Work out the finished part from the listing and answer in its coordinate system (mm). A direction names the side the tool comes from. Give positions to 0.01 mm unless a question says otherwise; leave off trailing zeros. Loops run counter-clockwise (first coordinate to the right, second up) from the corner with the lowest first, then second, coordinate; pieces in that order, holes last. Notation, with made-up numbers: (-38.75, 42) - (12.25, 42) arc R10 ccw to (12.25, 56) - close; hole circle Ø10 at (74.5, 33.5). An arc over 180 degrees is marked (long way). Use CSV: the item, a comma, the result in double quotes.
from build123d import *

# Parameters (mm, degrees)
F1_DEPTH = 600
F2_R     = 80
F3_DEPTH = 1321.7481718788
F5_DEPTH = 200.001
F6_DEPTH = 200.001


# Not quite as in the source:
# - a feature names something its author has since deleted; it is built from what else it names


with BuildPart() as f1:
    # F0 (on Front) → F1 (new body)
    with BuildSketch(Plane.XZ):
        with BuildLine():
            Line((506.8030357361, -100), (506.8030357361, 300))
            Line((506.8030357361, 300), (292.5279319286, 300))
            ThreePointArc((292.5279319286, 300), (-7.4720680714, 0), (-307.4720680714, 300))
            Line((-307.4720680714, 300), (-521.7471718788, 300))
            Line((-521.7471718788, 300), (-521.7471718788, -100))
            Line((-521.7471718788, -100), (-800, -100))
            Line((-800, -100), (-800, -300))
            Line((-800, -300), (800, -300))
            Line((800, -300), (800, -100))
            Line((800, -100), (506.8030357361, -100))
        make_face()
    extrude(amount=F1_DEPTH)

    # F2 (on face) → F3 (cut, through all)
    with BuildSketch(Plane(origin=(-521.7471718788, 0, 0), x_dir=(0, -1, 0), z_dir=(-1, 0, 0))):
        with Locations((287.7135872841, 150)):
            Circle(F2_R)
    extrude(amount=-F3_DEPTH, mode=Mode.SUBTRACT)

    # F4 (on face) → F5 (cut, through all)
    with BuildSketch(Plane.XY.offset(-100)):
        with BuildLine():
            Line((-610.4801893234, -509.8910629749), (-610.4801893234, -165.6369864941))
            Line((-610.4801893234, -165.6369864941), (-616.1602163315, -165.6369864941))
            ThreePointArc((-616.1602163315, -165.6369864941), (-676.1602163315, -105.6369864941), (-736.1602163315, -165.6369864941))
            Line((-736.1602163315, -165.6369864941), (-741.8402433395, -165.6369864941))
            Line((-741.8402433395, -165.6369864941), (-741.8402433395, -509.8910629749))
            Line((-741.8402433395, -509.8910629749), (-736.1602163315, -509.8910629749))
            ThreePointArc((-736.1602163315, -509.8910629749), (-676.1602163315, -569.8910629749), (-616.1602163315, -509.8910629749))
            Line((-616.1602163315, -509.8910629749), (-610.4801893234, -509.8910629749))
        make_face()
        with BuildLine():
            Line((704.2353129387, -496.3020980358), (712.1801376343, -496.3020980358))
            Line((712.1801376343, -496.3020980358), (712.1801376343, -165.6369864941))
            Line((712.1801376343, -165.6369864941), (704.2353129387, -165.6369864941))
            ThreePointArc((704.2353129387, -165.6369864941), (644.2353129387, -105.6369864941), (584.2353129387, -165.6369864941))
            Line((584.2353129387, -165.6369864941), (576.2904882431, -165.6369864941))
            Line((576.2904882431, -165.6369864941), (576.2904882431, -496.3020980358))
            Line((576.2904882431, -496.3020980358), (584.2353129387, -496.3020980358))
            ThreePointArc((584.2353129387, -496.3020980358), (644.2353129387, -556.3020980358), (704.2353129387, -496.3020980358))
        make_face()
    extrude(amount=-F5_DEPTH, mode=Mode.SUBTRACT)

    # F4 (on face) → F6 (cut, through all)
    with BuildSketch(Plane.XY.offset(-100)):
        with BuildLine():
            Line((-610.4801893234, -509.8910629749), (-610.4801893234, -165.6369864941))
            Line((-610.4801893234, -165.6369864941), (-616.1602163315, -165.6369864941))
            ThreePointArc((-616.1602163315, -165.6369864941), (-676.1602163315, -105.6369864941), (-736.1602163315, -165.6369864941))
            Line((-736.1602163315, -165.6369864941), (-741.8402433395, -165.6369864941))
            Line((-741.8402433395, -165.6369864941), (-741.8402433395, -509.8910629749))
            Line((-741.8402433395, -509.8910629749), (-736.1602163315, -509.8910629749))
            ThreePointArc((-736.1602163315, -509.8910629749), (-676.1602163315, -569.8910629749), (-616.1602163315, -509.8910629749))
            Line((-616.1602163315, -509.8910629749), (-610.4801893234, -509.8910629749))
        make_face()
        with BuildLine():
            Line((704.2353129387, -496.3020980358), (712.1801376343, -496.3020980358))
            Line((712.1801376343, -496.3020980358), (712.1801376343, -165.6369864941))
            Line((712.1801376343, -165.6369864941), (704.2353129387, -165.6369864941))
            ThreePointArc((704.2353129387, -165.6369864941), (644.2353129387, -105.6369864941), (584.2353129387, -165.6369864941))
            Line((584.2353129387, -165.6369864941), (576.2904882431, -165.6369864941))
            Line((576.2904882431, -165.6369864941), (576.2904882431, -496.3020980358))
            Line((576.2904882431, -496.3020980358), (584.2353129387, -496.3020980358))
            ThreePointArc((584.2353129387, -496.3020980358), (644.2353129387, -556.3020980358), (704.2353129387, -496.3020980358))
        make_face()
    extrude(amount=-F6_DEPTH, mode=Mode.SUBTRACT)


solid = f1.part
Item 1: A cutting plane is placed at A-A on y = -181.5. Determine the outline of the cut face in (x, z), and give its area (3 significant figures).
Determined:
outline,"(-800, -300) - (-741.84, -300) - (-741.84, -100) - (-800, -100) - close; (-610.48, -300) - (576.29, -300) - (576.29, -100) - (506.8, -100) - (506.8, 300) - (292.53, 300) arc R300 cw to (-307.47, 300) - (-521.75, 300) - (-521.75, -100) - (-610.48, -100) - close; (712.18, -300) - (800, -300) - (800, -100) - (712.18, -100) - close"
area,"537,000 mm²"
Item 2: A cutting plane is placed at C-C on z = -151. Determine the outline of the cut face in (x, y), and give its area (3 significant figures).
Determined:
outline,"(-800, -600) - (800, -600) - (800, 0) - (-800, 0) - close; hole (-741.84, -509.89) - (-736.16, -509.89) arc R60 ccw to (-616.16, -509.89) - (-610.48, -509.89) - (-610.48, -165.64) - (-616.16, -165.64) arc R60 ccw to (-736.16, -165.64) - (-741.84, -165.64) - close; hole (576.29, -496.3) - (584.24, -496.3) arc R60 ccw to (704.24, -496.3) - (712.18, -496.3) - (712.18, -165.64) - (704.24, -165.64) arc R60 ccw to (584.24, -165.64) - (576.29, -165.64) - close"
area,"847,000 mm²"
Item 3: A cutting plane is placed at D-D on y = -265.5. Determine the outline of the cut face in (x, z), and give its area (3 significant figures).
Determined:
outline,"(-800, -300) - (-741.84, -300) - (-741.84, -100) - (-800, -100) - close; (-610.48, -300) - (576.29, -300) - (576.29, -100) - (506.8, -100) - (506.8, 73.15) - (188.84, 73.15) arc R300 cw to (-203.78, 73.15) - (-521.75, 73.15) - (-521.75, -100) - (-610.48, -100) - close; (-521.75, 226.85) - (-298.42, 226.85) arc R300 cw to (-307.47, 300) - (-521.75, 300) - close; (283.47, 226.85) - (506.8, 226.85) - (506.8, 300) - (292.53, 300) arc R300 cw to start; (712.18, -300) - (800, -300) - (800, -100) - (712.18, -100) - close"
area,"457,000 mm²"
Item 4: A cutting plane is placed at B-B on x = -322. Determine the outline of the cut face in (y, z).
Determined:
outline,"(-600, -300) - (0, -300) - (0, 300) - (-600, 300) - close; hole circle Ø160 at (-287.71, 150)"
Item 5: Find the intervals of material crossed by line 1 (Y direction, x = -329.5, z = 150); line 2 (X direction, y = -526, z = -156); line 3 (X direction, y = -247.5, z = 259), in increasing order.
Determined:
line 1,"y = -600 to -367.71, -207.71 to 0"
line 2,"x = -800 to -733.96, -618.36 to 592.1, 696.37 to 800"
line 3,"x = -521.75 to -304.66, 289.71 to 506.8"
Item 6: Given P1, Ø4, axis at y = -425.5, z = 190.5, coming from the -X side; P2, Ø1, axis at x = 269, y = -331.5, coming from the +Z side; P3, Ø12, axis at x = -110.5, y = -266, coming from the +Z side, each flat-ended and moving along its own axis, determine where each tip first touches the part or whether it passes through.
Determined:
P1,"stops at x = -521.75"
P2,"stops at z = 83.38"
P3,"stops at z = 20.51"
Item 7: The mould has two halves that part along Y. Classify faces 5 (the cylindrical face through (379.301, -270.371, 71.902)), 6 (the flat face through (-11, -600, -129)), 7 (the flat face through (-597, -296, -100)): pulls with the +Y half, pulls with the -Y half, needs draft (parallel to the pull), parting line crosses it, or undercut.
Determined:
face 5,"undercut"
face 6,"pulls with the -Y half"
face 7,"needs draft"
Item 8: For faces 1 (the flat face through (576.29, -329, -199)), 2 (the flat face through (-521.747, -296, 58)), 3 (the flat face through (506.803, -296, 53)), 4 (the flat face through (401, -296, 300)), determine the directions among +Z, -Z, +X, -X, +Y, -Y from which every point of the face is accessible in a straight line to the end or side of a thin tool.
Determined:
face 1,"+Z, -Z"
face 2,"+Z, -X, +Y, -Y"
face 3,"+Z, +X, +Y, -Y"
face 4,"+Z, +X, -X, +Y, -Y"
